The listing builds one solid part. Answer for the finished solid, in the listing's coordinates (mm). Face numbers are marked on the shaded views. A direction names the side the tool comes from. Round coordinates to 2 decimals unless told otherwise and drop trailing zeros. Write each loop counter-clockwise with the first axis right and the second up, starting at its lowest first coordinate (ties: lowest second). Pieces come first, ordered by that corner, then holes. Notation, with made-up numbers: M -11,62 L 36,62 A13 ccw 36,83 Z; hole C 64,1.25 d5. An arc over 180 degrees is marked long. Write each question's results on one line, items separated by ' | '.
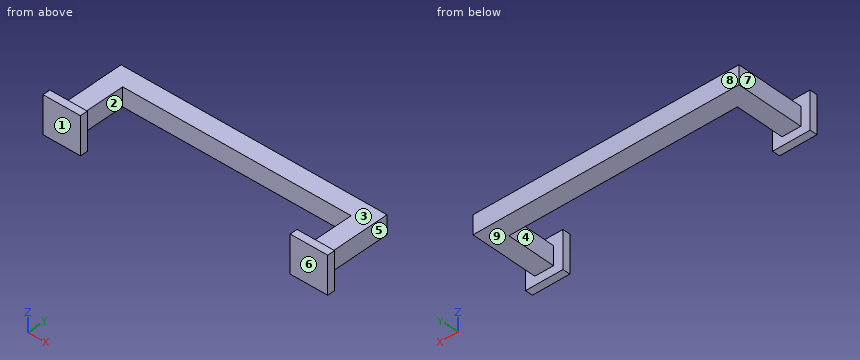
from build123d import *

# Parameters (mm, degrees)
PAD_DEPTH           = 2.5
SKETCH002_W         = 10
SKETCH002_H         = 10
PAD001_DEPTH        = 2
LINEARPATTERN_COUNT = 2
LINEARPATTERN_PITCH = 66


with BuildPart() as part:
    # Sketch001 → Pad (new body, symmetric)
    with BuildSketch(Plane.XY):
        Polygon((-35.5, 0), (-35.5, 20), (35.5, 20), (35.5, 0), (30.5, 0), (30.5, 15), (-30.5, 15), (-30.5, 0), align=None)
    extrude(amount=PAD_DEPTH, both=True)

    # Sketch002 (on Face4 of Pad) → Pad001 (join)
    with BuildSketch(Plane.XZ):
        with Locations((33, 0.228973)):
            Rectangle(SKETCH002_W, SKETCH002_H)
    pad001 = extrude(amount=-PAD001_DEPTH)

    # LinearPattern: Pad001 ×2
    with Locations(*[(-i * LINEARPATTERN_PITCH, 0, 0) for i in range(1, LINEARPATTERN_COUNT)]):
        add(pad001)


solid = part.part
1) A tool of negligible diameter and unlimited length cuts with its end or side. For the marked faces 5, 6, 7, 8 and 9, from which of +Z, -Z, +X, -X, +Y, -Y can it reach the whole face along a straight path? Write none if from no direction.
Return value:
face 5: +Z, -Z, +X, +Y | face 6: +Z, -Z, +X, -X, -Y | face 7: +Z, -Z, -X, +Y | face 8: +Z, -Z, +X, -X, +Y | face 9: -Z, +X, -X, +Y
2) The mould has two halves that part along Y. Classify the marked faces 1, 2, 3 and 4: +Y half, -Y half, draft (parallel to the pull), parting line (faces both ways), or undercut.
Return value:
face 1: -Y half | face 2: undercut | face 3: draft | face 4: undercut
3) Section D-D (x = -19.5) is taken. Determine the outline of the cut face in (y, z).
Return value:
outline: M 15,-2.5 L 20,-2.5 L 20,2.5 L 15,2.5 Z
4) Section A-A (y = 6.5) is taken. Determine the outline of the cut face in (x, z).
Return value:
outline: M -35.5,-2.5 L -30.5,-2.5 L -30.5,2.5 L -35.5,2.5 Z; M 30.5,-2.5 L 35.5,-2.5 L 35.5,2.5 L 30.5,2.5 Z
5) Each of these flat-tipped pins is pushed along its axis until it touches: pin 1 (5.5 mm diameter, centred on y = 11.5, z = 0, fed in from -X); pin 2 (1.5 mm diameter, centred on x = -14, y = 16.5, fed in from +Z); pin 3 (4 mm diameter, centred on y = 12.5, z = 4, fed in from +X); pin 4 (5.5 mm diameter, centred on x = 13.5, y = 10.5, fed in from -Z). Where does it stop, or does it pass through?
Return value:
pin 1: x = -35.5 | pin 2: z = 2.5 | pin 3: x = 35.5 | pin 4: through
6) Section B-B (z = 4.5) is taken. Determine the outline of the cut face in (x, y), then the cut area to 3 significant figures.
Return value:
outline: M -38,0 L -28,0 L -28,2 L -38,2 Z; M 28,0 L 38,0 L 38,2 L 28,2 Z | area: 40.0 mm²
7) Find the intervals of material crossed by line 1 (X direction, y = 9, z = -1.25); line 2 (Y direction, x = 28.5, z = 1.5); line 3 (Z direction, x = -7, y = 19), in increasing order.
Return value:
line 1: -35.5 to -30.5, 30.5 to 35.5 | line 2: 0 to 2, 15 to 20 | line 3: -2.5 to 2.5
8) Section C-C (z = 0) is taken. Determine the outline of the cut face in (x, y), then the cut area to 3 significant figures.
Return value:
outline: M -38,0 L -28,0 L -28,2 L -30.5,2 L -30.5,15 L 30.5,15 L 30.5,2 L 28,2 L 28,0 L 38,0 L 38,2 L 35.5,2 L 35.5,20 L -35.5,20 L -35.5,2 L -38,2 Z | area: 525 mm²
